Autodesk Inventor part; units mm, degrees
ref_plane "YZ Plane" through (0, 0, 0) normal (1, 0, 0) x (0, 1, 0)
ref_plane "XZ Plane" through (0, 0, 0) normal (0, 1, 0) x (-1, 0, 0)
ref_plane "XY Plane" through (0, 0, 0) normal (0, 0, 1) x (1, 0, 0)
sketch "Sketch1" plane through (0, 0, 0) normal (0, 0, 1) x (1, 0, 0)
  circle A0 centre (0, 0) radius 20.9
  circle A1 centre (0, 0) radius 13
  dimension "d0" = 41.8
  dimension "d1" = 26
extrude "Extrusion1" add sketch "Sketch1" along normal mid plane 23.368
sketch "Sketch2" plane through (0, 0, 11.684) normal (0, 0, 1) x (1, 0, 0)
  circle A0 centre (0, 0) radius 13
  point P0 (0, 17.5)
  dimension "d4" = 17.5
hole "Hole1" at (0, 17.5, 11.684) direction (0, 0, -1) diameter 3.5 end through all
pattern_circular "Circular Pattern1" count 4 over 360 about axis through (0, 0, 0) along (0, 0, 1) of "Hole1"
sketch "Sketch3" plane through (0, 0, 11.684) normal (0, 0, 1) x (1, 0, 0)
  circle A0 centre (0, 0) radius 13
  circle A1 centre (0, 0) radius 20.9
  circle A2 centre (0, 0) radius 14.5
  dimension "d15" = 29
extrude "Extrusion2" cut sketch "Sketch3" against normal blind 1.75 contours A2
mirror "Mirror1" about plane through (0, 0, 0) normal (0, 0, 1) of "Extrusion2"
properties part number "BB1-RingGear" material "Aluminum-6061"
Could you check a few things on this model? Use its own coordinates, in mm. A direction names the side the tool comes from. Give positions to 0.01 mm unless a question says otherwise; leave off trailing zeros. Order: outer loops, then holes, each group sorted by start corner. A loop starts at its lowest first (then second) coordinate and runs counter-clockwise, first axis right, second up.
Q1. Suppose I cut it at D-D, the plane y = -11.5. Write out the boundary of the cut face in (x, z).
Q2. If I drill on line 1 along Y through (x, z) = (1.5, -8.5); line 2 along Y through (x, z) = (-1.5, 10.25); line 3 along Y through (x, z) = (16, 5.5), over which ranges is the centre line in solid material (lowest first)?
Q3. For faces 1 (the cylindrical face through (6.691, -12.864, 10.821)), 2 (the cylindrical face through (0.08, -19.25, -0.16)), 3 (the flat face through (9, 10, -9.934)), which set-ups out of +Z, -Z, +X, -X, +Y, -Y let a thin tool reach every point of the face, with its end or its side?
Q4. Suppose I cut it at C-C, the plane z = 1.5. Write out the boundary of the cut face in (x, y).
Q5. Suppose I cut it at A-A, the plane y = 0. Write out the boundary of the cut face in (x, z), and give its area (3 significant figures).
Q6. We'd pull the mould along X, two halves only. Please class faces 4 (the cylindrical face through (-15.4, -14.13, -0.16)), 5 (the cylindrical face through (19.25, 0.08, -0.16)), 6 (the flat face through (-9, 10, 9.934)), 7 (the flat face through (14, 5, 11.684)): +X half, -X half, draft (parallel to the pull), parting line (faces both ways), or undercut.
Q7. I'm going to push flat-ended pins straight in: P1, Ø1.5, axis at y = -2, z = -8.5, coming from the +X side; P2, Ø4.5, axis at x = 0, y = -17.5, coming from the -Z side; P3, Ø12, axis at y = 8, z = -2, coming from the -X side; P4, Ø1, axis at y = 6.5, z = -8, coming from the -X side. Where does each tip first touch, or does it pass through?
Solution:
1. outline: (-17.45, -11.68) - (-8.83, -11.68) - (-8.83, -9.93) - (-6.06, -9.93) - (-6.06, 9.93) - (-8.83, 9.93) - (-8.83, 11.68) - (-17.45, 11.68) - close; (6.06, -9.93) - (8.83, -9.93) - (8.83, -11.68) - (17.45, -11.68) - (17.45, 11.68) - (8.83, 11.68) - (8.83, 9.93) - (6.06, 9.93) - close
2. line 1: y = -20.85 to -18.4, -16.6 to -12.91, 12.91 to 16.6, 18.4 to 20.85
2. line 2: y = -20.85 to -18.4, -16.6 to -14.42, 14.42 to 16.6, 18.4 to 20.85
2. line 3: y = -13.45 to -0.9, 0.9 to 13.45
3. face 1: +Z
3. face 2: +Z, -Z
3. face 3: -Z
4. outline: circle Ø41.8 at (0, 0); hole circle Ø3.5 at (-17.5, 0); hole circle Ø26 at (0, 0); hole circle Ø3.5 at (0, -17.5); hole circle Ø3.5 at (0, 17.5); hole circle Ø3.5 at (17.5, 0)
5. outline: (-20.9, -11.68) - (-19.25, -11.68) - (-19.25, 11.68) - (-20.9, 11.68) - close; (-15.75, -11.68) - (-14.5, -11.68) - (-14.5, -9.93) - (-13, -9.93) - (-13, 9.93) - (-14.5, 9.93) - (-14.5, 11.68) - (-15.75, 11.68) - close; (13, -9.93) - (14.5, -9.93) - (14.5, -11.68) - (15.75, -11.68) - (15.75, 11.68) - (14.5, 11.68) - (14.5, 9.93) - (13, 9.93) - close; (19.25, -11.68) - (20.9, -11.68) - (20.9, 11.68) - (19.25, 11.68) - close
5. area: 195 mm2
6. face 4: parting line
6. face 5: undercut
6. face 6: undercut
6. face 7: draft
7. P1: stops at x = 20.86
7. P2: stops at z = -11.68
7. P3: stops at x = -20.8
7. P4: stops at x = -20.02
